Autodesk Inventor part; units mm, degrees
ref_plane "YZ Plane" through (0, 0, 0) normal (1, 0, 0) x (0, 1, 0)
ref_plane "XZ Plane" through (0, 0, 0) normal (0, 1, 0) x (-1, 0, 0)
ref_plane "XY Plane" through (0, 0, 0) normal (0, 0, 1) x (1, 0, 0)
sketch "Sketch1" plane through (0, 0, 0) normal (0, 0, 1) x (1, 0, 0)
  line L0 (-21, 22.5) -> (21, 22.5)
  line L1 (21, 22.5) -> (21, -22.5)
  line L2 (21, -22.5) -> (-21, -22.5)
  line L3 (-21, -22.5) -> (-21, 22.5)
  line L4 (-21, 22.5) -> (21, -22.5) construction
  line L5 (21, 22.5) -> (-21, -22.5) construction
  line L6 (-6, 19.5) -> (-6, -19.5) construction
  line L7 (-21, 0) -> (21, 0) construction
  arc A0 (-8.2361, 21.5) -> (-3.7639, 21.5) centre (-6, 19.5) ccw
  line L8 (20.0667, -21.5) -> (-20.0667, -21.5)
  line L9 (-20.0667, -21.5) -> (-20.0667, 21.5)
  line L10 (-20.0667, 21.5) -> (20.0667, 21.5)
  line L11 (20.0667, 21.5) -> (20.0667, -21.5)
  line L12 (20.0667, -21.5) -> (-20.0667, 21.5) construction
  line L13 (-20.0667, -21.5) -> (20.0667, 21.5) construction
  arc A1 (-3.7639, -21.5) -> (-8.2361, -21.5) centre (-6, -19.5) ccw
  point P0 (0, 0)
  point P1 (-8.2361, -21.5)
  point P2 (-3.7639, -21.5)
  dimension "d0" = 42
  dimension "d1" = 45
  dimension "d2" = 15
  dimension "d3" = 39
  dimension "d6" = 1
  dimension "d7" = 6
extrude "Extrusion1" add sketch "Sketch1" against normal blind 1.6 contours L0 L1 L2 L3 | L10 A0 | A0 L10 L11 L8 A1 L9 | A1 L8
extrude "Extrusion2" add sketch "Sketch1" along normal blind 15 contours A0 L10 L11 L8 A1 L9
fillet "Fillet1" radius 2 16 edges at (-3.7639, 21.5, 7.5) (-8.2361, 21.5, 7.5) (-3.7639, -21.5, 7.5) (-8.2361, -21.5, 7.5) (-20.0667, 21.5, 7.5) (-20.0667, -21.5, 7.5) (20.0667, -21.5, 7.5) (20.0667, 21.5, 7.5) (20.0667, 0, 15) (8.1514, 21.5, 15) (-14.1514, 21.5, 15) (-6, 16.5, 15) (-20.0667, 0, 15) (-14.1514, -21.5, 15) (-6, -16.5, 15) (8.1514, -21.5, 15)
hole "Hole1" at (-6, 19.5, 0) at (-6, -19.5, 0) direction (0, 0, -1) diameter 3.5 end through all
properties part number "AKI.DAC-U2704 REV.C" material "Acetal Resin, Black"
Read the model definition and answer for the solid it produces. Units are mm, in the model's axes. A direction names the side the tool comes from. Give positions to 0.01 mm unless a question says otherwise; leave off trailing zeros. Write each loop counter-clockwise with the first axis right and the second up, starting at its lowest first coordinate (ties: lowest second). Pieces come first, ordered by that corner, then holes. Notation, with made-up numbers: (21, -19.5) -> (45, -19.5) arc R10 cw to (45, -12.5) -> close; hole circle Ø10 at (19, 89). An arc over 180 degrees is marked (long way). Answer as a JSON object with one key per item and string values. Group by question number.
1) Find section C-C (y = 4). Write down the section's boundary in (x, z).
2) Find section D-D (x = 5.5). Write down the section's boundary in (y, z), and give its area (3 significant figures).
3) Find section A-A (x = -6). Write down the section's boundary in (y, z).
4) The mould has two halves that part along X. Classify faces 5 (the flat face through (8, 21.5, 6)), 6 (the flat face through (21, 0, -1)), 7 (the cylindrical face through (-4.94, -18.11, -0.81)), 8 (the cylindrical face through (-19.496, 0.273, 14.399)): +X half, -X half, draft (parallel to the pull), parting line (faces both ways), or undercut.
5) A tool of negligible diameter and unlimited length cuts with its end or side. For faces 1 (the cylindrical face through (-9.6, -20.93, 6.59)), 2 (the cylindrical face through (-9.57, 20.9, 6.59)), 3 (the flat face through (20.067, 0, 6)), 4 (the flat face through (-5, 17, 0)), from which of +Z, -Z, +X, -X, +Y, -Y can it reach the whole face along a straight path? Write none if from no direction.
6) Each of these flat-tipped pins is pushed along its axis until it touches: P1, Ø5.5, axis at x = -15, z = 9.5, coming from the +Y side; P2, Ø4, axis at x = 6, z = 4, coming from the -Y side; P3, Ø1, axis at y = -9, z = 5.5, coming from the -X side. Where does it stop, or does it pass through?
7) Consider L1, parallel to Y at x = -6, z = -0.4; L2, parallel to X at y = -19.5, z = -0.25; L3, parallel to Y at x = -17, z = 11.75. Determine where each line is inside the solid, lowest interval first. Write a range as from..to.
8) Find section B-B (z = 11.5). Write down the section's boundary in (x, y).
Values follow:
{
 "1": {"outline": "(-21, -1.6) -> (21, -1.6) -> (21, 0) -> (20.07, 0) -> (20.07, 13) arc R2 ccw to (18.07, 15) -> (-18.07, 15) arc R2 ccw to (-20.07, 13) -> (-20.07, 0) -> (-21, 0) -> close"},
 "2": {"outline": "(-22.5, -1.6) -> (22.5, -1.6) -> (22.5, 0) -> (21.5, 0) -> (21.5, 13) arc R2 ccw to (19.5, 15) -> (-19.5, 15) arc R2 ccw to (-21.5, 13) -> (-21.5, 0) -> (-22.5, 0) -> close", "area": "715 mm2"},
 "3": {"outline": "(-22.5, -1.6) -> (-21.25, -1.6) -> (-21.25, 0) -> (-22.5, 0) -> close; (-17.75, -1.6) -> (17.75, -1.6) -> (17.75, 0) -> (16.5, 0) -> (16.5, 13) arc R2 ccw to (14.5, 15) -> (-14.5, 15) arc R2 ccw to (-16.5, 13) -> (-16.5, 0) -> (-17.75, 0) -> close; (21.25, -1.6) -> (22.5, -1.6) -> (22.5, 0) -> (21.25, 0) -> close"},
 "4": {"face 5": "draft", "face 6": "+X half", "face 7": "undercut", "face 8": "-X half"},
 "5": {"face 1": "+Z, -Y", "face 2": "+Z, +Y", "face 3": "+Z, +X, +Y, -Y", "face 4": "+Z"},
 "6": {"P1": "stops at y = 21.5", "P2": "stops at y = -21.5", "P3": "stops at x = -20.07"},
 "7": {"L1": "y = -22.5..-21.25, -17.75..17.75, 21.25..22.5", "L2": "x = -21..-7.75, -4.25..21", "L3": "y = -21.5..21.5"},
 "8": {"outline": "(-20.07, -19.5) arc R2 ccw to (-18.07, -21.5) -> (-11, -21.5) arc R2 ccw to (-9, -19.5) arc R3 cw to (-3, -19.5) arc R2 ccw to (-1, -21.5) -> (18.07, -21.5) arc R2 ccw to (20.07, -19.5) -> (20.07, 19.5) arc R2 ccw to (18.07, 21.5) -> (-1, 21.5) arc R2 ccw to (-3, 19.5) arc R3 cw to (-9, 19.5) arc R2 ccw to (-11, 21.5) -> (-18.07, 21.5) arc R2 ccw to (-20.07, 19.5) -> close"}
}
